The listing builds one solid part. Answer for the finished solid, in the listing's coordinates (mm). Give positions to 0.01 mm unless a question says otherwise; leave off trailing zeros. Order: outer loops, then holes, each group sorted by start corner. A loop starts at its lowest first (then second) coordinate and runs counter-clockwise, first axis right, second up. Notation, with made-up numbers: (-26.5, 9.5) -> (18.5, 9.5) arc R8 cw to (18.5, 23.5) -> close; hole circle Ø2 at (65.25, -20.75). An arc over 180 degrees is marked (long way). Answer as a JSON object with one key per item and string values. Group by question number.
```python
from build123d import *

# Parameters (mm, degrees)
ESQUISSE1_W             = 80
ESQUISSE1_H             = 80
EXTRUSION1_DEPTH        = 1
CONG_1_R                = 5
ESQUISSE2_W             = 14
ESQUISSE2_H             = 14
ENL_V_MAT_EXTRU_1_DEPTH = 2


with BuildPart() as part:
    # Esquisse1 → Extrusion1 (new body)
    with BuildSketch(Plane(origin=(0, 0, 0), x_dir=(1, 0, 0), z_dir=(0, 1, 0))):
        with Locations((40, 40)):
            Rectangle(ESQUISSE1_W, ESQUISSE1_H)
    extrude(amount=EXTRUSION1_DEPTH)

    # Congé1
    cong_1_edges = [part.edges().sort_by_distance(p)[0] for p in [
        (0, 0.5, -80),
        (80, 0.5, -80),
        (80, 0.5, 0),
        (0, 0.5, 0),
    ]]
    fillet(cong_1_edges, radius=CONG_1_R)

    # Esquisse2 → Enlèv. mat.-Extru.1 (cut, through all)
    with BuildSketch(Plane(origin=(0, 1, 0), x_dir=(1, 0, 0), z_dir=(0, 1, 0))):
        with Locations((40, 40)):
            Rectangle(ESQUISSE2_W, ESQUISSE2_H)
    extrude(amount=-ENL_V_MAT_EXTRU_1_DEPTH, mode=Mode.SUBTRACT)


solid = part.part
```
(1) A cutting plane is placed at C-C (y = 0.8). Determine the outline of the cut face in (x, z), and give its area (3 significant figures).
(2) Find the intervals of material crossed by line 1 along X through (y, z) = (0.1, -40.5); line 2 along Z through (x, y) = (36, 0.65), in increasing order. Write a range as [from, to].
(3) A cutting plane is placed at B-B (x = 34.5). Determine the outline of the cut face in (y, z), and give its area (3 significant figures).
(4) A cutting plane is placed at A-A (z = -36.5). Determine the outline of the cut face in (x, y), and give its area (3 significant figures).
Check sheet entries:
{
 "1": {"outline": "(0, -75) arc R5 ccw to (5, -80) -> (75, -80) arc R5 ccw to (80, -75) -> (80, -5) arc R5 ccw to (75, 0) -> (5, 0) arc R5 ccw to (0, -5) -> close; hole (33, -47) -> (47, -47) -> (47, -33) -> (33, -33) -> close", "area": "6,180 mm2"},
 "2": {"line 1": "x = [0, 33], [47, 80]", "line 2": "z = [-80, -47], [-33, 0]"},
 "3": {"outline": "(0, -80) -> (1, -80) -> (1, -47) -> (0, -47) -> close; (0, -33) -> (1, -33) -> (1, 0) -> (0, 0) -> close", "area": "66.0 mm2"},
 "4": {"outline": "(0, 0) -> (33, 0) -> (33, 1) -> (0, 1) -> close; (47, 0) -> (80, 0) -> (80, 1) -> (47, 1) -> close", "area": "66.0 mm2"}
}
